For this review, take the finished solid that the model builds, in its own axes (mm). A direction names the side the tool comes from. Give positions to 0.01 mm unless a question says otherwise; leave off trailing zeros. Loops run counter-clockwise (first coordinate to the right, second up) from the corner with the lowest first, then second, coordinate; pieces in that order, holes last. Notation, with made-up numbers: (89.25, 73.25) -> (121.25, 73.25) arc R13 cw to (121.25, 88.25) -> close; hole circle Ø11 at (-16.5, 26). An arc over 180 degrees is marked (long way). Write each question's results on one line, items separated by ' | '. Start each with the question number.
```python
from build123d import *

# Parameters (mm, degrees)
BOSS_EXTRUDE1_DEPTH = 2
SKETCH4_R           = 1.5
CUT_EXTRUDE3_DEPTH  = 2
SKETCH6_R           = 35
CUT_EXTRUDE4_DEPTH  = 1
SKETCH7_R           = 11
SKETCH7_R_2         = 2.6
SKETCH7_R_3         = 8
CUT_EXTRUDE5_DEPTH  = 10


with BuildPart() as part:
    # Sketch1 → Boss-Extrude1 (new body)
    with BuildSketch(Plane.XY):
        with BuildLine():
            Line((21.520746486, 52.119258472), (15.256667967, 42.372162038))
            Line((15.256667967, 42.372162038), (32.20522538, 31.479985569))
            Line((32.20522538, 31.479985569), (38.4693039, 41.227082003))
            ThreePointArc((38.4693039, 41.227082003), (40.698070229, 42.590620718), (43.150594208, 41.689641633))
            ThreePointArc((43.150594208, 41.689641633), (45.344974461, 39.291644037), (47.406271028, 36.778328771))
            ThreePointArc((47.406271028, 36.778328771), (47.949048893, 34.222545257), (46.282202516, 32.210516346))
            Line((46.282202516, 32.210516346), (35.742846148, 27.397353567))
            Line((35.742846148, 27.397353567), (44.112124759, 9.071189697))
            Line((44.112124759, 9.071189697), (54.651481127, 13.884352476))
            ThreePointArc((54.651481127, 13.884352476), (57.263623361, 13.826472187), (58.839711753, 11.742585779))
            ThreePointArc((58.839711753, 11.742585779), (59.389286513, 8.538890296), (59.764558712, 5.310133889))
            ThreePointArc((59.764558712, 5.310133889), (58.83941162, 2.86662411), (56.349386262, 2.075162869))
            Line((56.349386262, 2.075162869), (44.880923224, 3.724078919))
            Line((44.880923224, 3.724078919), (42.013736207, -16.217644809))
            Line((42.013736207, -16.217644809), (53.482199245, -17.86656086))
            ThreePointArc((53.482199245, -17.86656086), (55.648380681, -19.32748357), (55.847636558, -21.93265809))
            ThreePointArc((55.847636558, -21.93265809), (54.577919721, -24.92490078), (53.148021281, -27.843990983))
            ThreePointArc((53.148021281, -27.843990983), (51.048676897, -29.399429937), (48.526038015, -28.719040157))
            Line((48.526038015, -28.719040157), (39.76962429, -21.131564473))
            Line((39.76962429, -21.131564473), (26.576283265, -36.357491677))
            Line((26.576283265, -36.357491677), (35.33269699, -43.944967362))
            ThreePointArc((35.33269699, -43.944967362), (36.365170327, -46.345099856), (35.124331356, -48.644437984))
            ThreePointArc((35.124331356, -48.644437984), (32.438449047, -50.47521197), (29.657362619, -52.157845455))
            ThreePointArc((29.657362619, -52.157845455), (27.050347952, -52.331372705), (25.296015568, -50.395150852))
            Line((25.296015568, -50.395150852), (22.031750643, -39.278085453))
            Line((22.031750643, -39.278085453), (2.701048165, -44.954091828))
            Line((2.701048165, -44.954091828), (5.96531309, -56.071157227))
            ThreePointArc((5.96531309, -56.071157227), (5.536275339, -58.648474396), (3.249299125, -59.911952524))
            ThreePointArc((3.249299125, -59.911952524), (0, -60), (-3.249299125, -59.911952524))
            ThreePointArc((-3.249299125, -59.911952524), (-5.536275339, -58.648474396), (-5.96531309, -56.071157227))
            Line((-5.96531309, -56.071157227), (-2.701048165, -44.954091828))
            Line((-2.701048165, -44.954091828), (-22.031750643, -39.278085453))
            Line((-22.031750643, -39.278085453), (-25.296015568, -50.395150852))
            ThreePointArc((-25.296015568, -50.395150852), (-27.050347952, -52.331372705), (-29.657362619, -52.157845455))
            ThreePointArc((-29.657362619, -52.157845455), (-32.438449047, -50.47521197), (-35.124331356, -48.644437984))
            ThreePointArc((-35.124331356, -48.644437984), (-36.365170327, -46.345099856), (-35.33269699, -43.944967362))
            Line((-35.33269699, -43.944967362), (-26.576283265, -36.357491677))
            Line((-26.576283265, -36.357491677), (-39.76962429, -21.131564473))
            Line((-39.76962429, -21.131564473), (-48.526038015, -28.719040157))
            ThreePointArc((-48.526038015, -28.719040157), (-51.048676897, -29.399429937), (-53.148021281, -27.843990983))
            ThreePointArc((-53.148021281, -27.843990983), (-54.577919721, -24.92490078), (-55.847636558, -21.93265809))
            ThreePointArc((-55.847636558, -21.93265809), (-55.648380681, -19.32748357), (-53.482199245, -17.86656086))
            Line((-53.482199245, -17.86656086), (-42.013736207, -16.217644809))
            Line((-42.013736207, -16.217644809), (-44.880923224, 3.724078919))
            Line((-44.880923224, 3.724078919), (-56.349386262, 2.075162869))
            ThreePointArc((-56.349386262, 2.075162869), (-58.83941162, 2.86662411), (-59.764558712, 5.310133889))
            ThreePointArc((-59.764558712, 5.310133889), (-59.389286513, 8.538890296), (-58.839711753, 11.742585779))
            ThreePointArc((-58.839711753, 11.742585779), (-57.263623361, 13.826472187), (-54.651481127, 13.884352476))
            Line((-54.651481127, 13.884352476), (-44.112124759, 9.071189697))
            Line((-44.112124759, 9.071189697), (-35.742846148, 27.397353567))
            Line((-35.742846148, 27.397353567), (-46.282202516, 32.210516346))
            ThreePointArc((-46.282202516, 32.210516346), (-47.949048893, 34.222545257), (-47.406271028, 36.778328771))
            ThreePointArc((-47.406271028, 36.778328771), (-45.344974461, 39.291644037), (-43.150594208, 41.689641633))
            ThreePointArc((-43.150594208, 41.689641633), (-40.698070229, 42.590620718), (-38.4693039, 41.227082003))
            Line((-38.4693039, 41.227082003), (-32.20522538, 31.479985569))
            Line((-32.20522538, 31.479985569), (-15.256667967, 42.372162038))
            Line((-15.256667967, 42.372162038), (-21.520746486, 52.119258472))
            ThreePointArc((-21.520746486, 52.119258472), (-21.835201934, 54.713050089), (-19.99682725, 56.569664131))
            ThreePointArc((-19.99682725, 56.569664131), (-16.90395341, 57.569578417), (-13.76146789, 58.400530832))
            ThreePointArc((-13.76146789, 58.400530832), (-11.211167359, 57.832548102), (-10.073394495, 55.480504291))
            Line((-10.073394495, 55.480504291), (-10.073394495, 43.894108449))
            Line((-10.073394495, 43.894108449), (10.073394495, 43.894108449))
            Line((10.073394495, 43.894108449), (10.073394495, 55.480504291))
            ThreePointArc((10.073394495, 55.480504291), (11.211167359, 57.832548102), (13.76146789, 58.400530832))
            ThreePointArc((13.76146789, 58.400530832), (16.90395341, 57.569578417), (19.99682725, 56.569664131))
            ThreePointArc((19.99682725, 56.569664131), (21.835201934, 54.713050089), (21.520746486, 52.119258472))
        make_face()
    extrude(amount=BOSS_EXTRUDE1_DEPTH)

    # Sketch4 → Cut-Extrude3 (cut)
    with BuildSketch(Plane.XY.offset(2)):
        with Locations((-14.086627842, 47.974648681)):
            Circle(SKETCH4_R)
        with Locations((14.086627842, 47.974648681)):
            Circle(SKETCH4_R)
        with Locations((37.787478718, 32.743036697)):
            Circle(SKETCH4_R)
        with Locations((49.491072094, 7.115741914)):
            Circle(SKETCH4_R)
        with Locations((45.481599768, -20.77075065)):
            Circle(SKETCH4_R)
        with Locations((27.032040873, -42.062676642)):
            Circle(SKETCH4_R)
        with Locations((0, -50)):
            Circle(SKETCH4_R)
        with Locations((-27.032040873, -42.062676642)):
            Circle(SKETCH4_R)
        with Locations((-45.481599768, -20.77075065)):
            Circle(SKETCH4_R)
        with Locations((-49.491072094, 7.115741914)):
            Circle(SKETCH4_R)
        with Locations((-37.787478718, 32.743036697)):
            Circle(SKETCH4_R)
    extrude(amount=-CUT_EXTRUDE3_DEPTH, mode=Mode.SUBTRACT)

    # Sketch6 → Cut-Extrude4 (cut)
    with BuildSketch(Plane(origin=(0, 0, 0), x_dir=(-1, 0, 0), z_dir=(0, 0, -1))):
        Circle(SKETCH6_R)
    extrude(amount=-CUT_EXTRUDE4_DEPTH, mode=Mode.SUBTRACT)

    # Sketch7 → Cut-Extrude5 (cut)
    with BuildSketch(Plane(origin=(0, 0, 1), x_dir=(-1, 0, 0), z_dir=(0, 0, -1))):
        Circle(SKETCH7_R)
        with Locations((-6.691148225, 22.787958123)):
            Circle(SKETCH7_R_2)
        with Locations((-18.093350953, 17.251975287)):
            Circle(SKETCH7_R_3)
        with Locations((5.893973388, 24.295289208)):
            Circle(SKETCH7_R_3)
        with Locations((16.389376523, 17.188683405)):
            Circle(SKETCH7_R_2)
        with Locations((23.98732434, 7.043313921)):
            Circle(SKETCH7_R_3)
        with Locations((23.080524748, -5.599274718)):
            Circle(SKETCH7_R_2)
        with Locations((18.093350953, -17.251975287)):
            Circle(SKETCH7_R_3)
        with Locations((6.691148225, -22.787958123)):
            Circle(SKETCH7_R_2)
        with Locations((-5.893973388, -24.295289208)):
            Circle(SKETCH7_R_3)
        with Locations((-16.389376523, -17.188683405)):
            Circle(SKETCH7_R_2)
        with Locations((-23.98732434, -7.043313921)):
            Circle(SKETCH7_R_3)
        with Locations((-23.080524748, 5.599274718)):
            Circle(SKETCH7_R_2)
    extrude(amount=-CUT_EXTRUDE5_DEPTH, mode=Mode.SUBTRACT)


solid = part.part
```
1. Machinability: for faces 4 (the flat face through (-31.016, -40.204, 0.986)), 5 (the flat face through (-12.231, -42.156, 0.986)), 6 (the flat face through (8, 8, 1)), which of the approach directions +Z, -Z, +X, -X, +Y, -Y give a long, thin tool a straight path to every point of the face, cutting with its end or side? Answer none if there is none.
2. We need section A-A (x = 0). Write out the cut boundary in (y, z), plus the area to 3 significant figures.
3. For pin 1 Ø4 at (x, y) = (23.08, 5.6) entering from +Z; pin 2 Ø1 at (x, z) = (-20.5, 1.5) entering from -Y; pin 3 Ø8 at (x, y) = (21.5, -17.5) entering from -Z; pin 4 Ø1 at (x, z) = (4.5, 1.5) entering from +Y, all flat-tipped, find the tip position at first contact; note any pin that passes through.
4. Draft analysis for pull direction X (two halves, no side actions). For faces 1 (the cylindrical face through (-45.37, 39.26, 0.99)), 2 (the cylindrical face through (-44.05, -20.32, 1.01)), 3 (the flat face through (1, 13, 2)), state which applies: released by +X, released by -X, zero draft, split by the parting line, or undercut.
5. Wall thickness on L1, parallel to Y at x = 21.5, z = 1.1; L2, parallel to Y at x = 29.5, z = 0.2; L3, parallel to X at y = 39, z = 1.5: over which ranges is each line inside the solid? List them lowest first.
Response:
1) face 4: +Z, -Z, -X | face 5: +Z, -Z | face 6: -Z
2) outline: (-60, 0) -> (-51.5, 0) -> (-51.5, 2) -> (-60, 2) -> close; (-48.5, 0) -> (-35, 0) -> (-35, 1) -> (-29.7, 1) -> (-29.7, 2) -> (-48.5, 2) -> close; (-18.89, 1) -> (-11, 1) -> (-11, 2) -> (-18.89, 2) -> close; (11, 1) -> (18.89, 1) -> (18.89, 2) -> (11, 2) -> close; (29.7, 1) -> (35, 1) -> (35, 0) -> (43.89, 0) -> (43.89, 2) -> (29.7, 2) -> close | area: 88.2 mm2
3) pin 1: passes through | pin 2: stops at y = -39.87 | pin 3: stops at z = 1 | pin 4: stops at y = 43.89
4) face 1: released by -X | face 2: undercut | face 3: zero draft
5) L1: y = -39.43 to -14.65, 0.56 to 3.53, 7.66 to 10.01, 24.49 to 38.36, 52.09 to 55.39 | L2: y = -52.24 to -38.89, -32.98 to -18.83, 18.83 to 33.22 | L3: x = -45.6 to -37.04, -20.5 to 20.5, 37.04 to 45.6
